Here's how the part is built. I have some questions about the finished solid (model axes, mm). Face numbers are marked on the shaded views. A direction names the side the tool comes from. Give positions to 0.01 mm unless a question says otherwise; leave off trailing zeros. Loops run counter-clockwise (first coordinate to the right, second up) from the corner with the lowest first, then second, coordinate; pieces in that order, holes last. Notation, with made-up numbers: M 78,-20 L 101,-20 A21 ccw 101,-3 Z; hole C 33.5,33.5 d4. An arc over 180 degrees is marked long. Answer as CSV lines item,"result". Start each with the question number.
Item 1: I want a section at B-B on x = -22. List the corners of the cut face in (y, z) for me, plus the area to 3 significant figures.
Item 2: For the marked faces 1 and 2, which set-ups out of +Z, -Z, +X, -X, +Y, -Y let a thin tool reach every point of the face, with its end or its side?
Item 3: I want a section at A-A on z = 20. List the corners of the cut face in (x, y) for me.
Item 4: Will these pins go through, and if not, where does the flat tip stop? P1, Ø19, axis at y = -52, z = 14, coming from the -X side; P2, Ø10, axis at y = 74, z = 34, coming from the -X side; P3, Ø1.5, axis at x = -24, z = 34, coming from the -Y side; P4, Ø1, axis at x = -30, y = 95.5, coming from the -Z side.
Item 5: If I drill on line 1 along Y through (x, z) = (-32.5, 25.5); line 2 along X through (y, z) = (57, 13.5), over which ranges is the centre line in solid material (lowest first)? Write a range as from..to.
Item 6: I want a section at C-C on y = 46.5. List the corners of the cut face in (x, z) for me.
from build123d import *

# Parameters (mm, degrees)
F0_W     = 38.1
F0_H     = 215.9
F0_H_2   = 38.1
F0_W_2   = 63.5
F1_DEPTH = 38.1
F2_SIZE  = 12.7
F3_SIZE  = 31.75
F4_SIZE  = 6.35


with BuildPart() as f1:
    # F0 (on Top) → F1 (new body)
    with BuildSketch(Plane.XY):
        with Locations((0, -19.05)):
            Rectangle(F0_W, F0_H)
        with Locations((0, 107.95)):
            Rectangle(F0_W, F0_H_2)
        with Locations((-50.8, 107.95)):
            Rectangle(F0_W_2, F0_H_2)
    extrude(amount=F1_DEPTH)

    # F2
    f2_edges = [f1.edges().sort_by_distance(p)[0] for p in [
        (-19.05, 88.9, 19.05),
    ]]
    chamfer(f2_edges, length=F2_SIZE)

    # F3
    f3_edges = [f1.edges().sort_by_distance(p)[0] for p in [
        (19.05, 127, 19.05),
    ]]
    chamfer(f3_edges, length=F3_SIZE)

    # F4
    f4_edges = [f1.edges().sort_by_distance(p)[0] for p in [
        (-82.55, 88.9, 19.05),
        (-82.55, 127, 19.05),
    ]]
    chamfer(f4_edges, length=F4_SIZE)


solid = f1.part
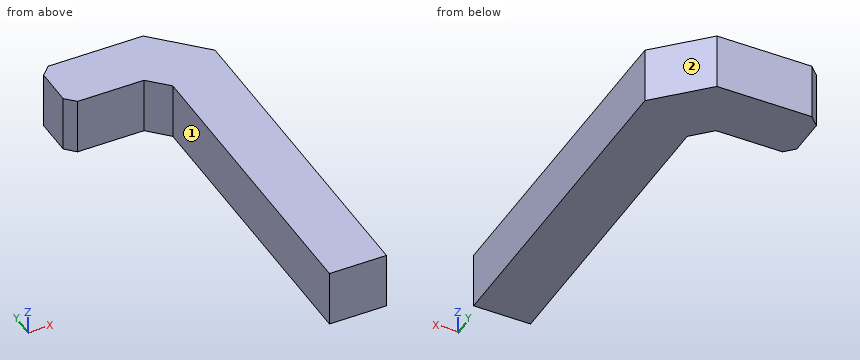
Result:
1,outline,"M 79.15,0 L 127,0 L 127,38.1 L 79.15,38.1 Z"
1,area,"1,820 mm^2"
2,face 1,"+Z, -Z, -X, -Y"
2,face 2,"+Z, -Z, +X, +Y"
3,outline,"M -82.55,95.25 L -76.2,88.9 L -31.75,88.9 L -19.05,76.2 L -19.05,-127 L 19.05,-127 L 19.05,95.25 L -12.7,127 L -76.2,127 L -82.55,120.65 Z"
4,P1,"x = -19.05"
4,P2,"x = -21.85"
4,P3,"y = 80.4"
4,P4,"z = 0"
5,line 1,"88.9..127"
5,line 2,"-19.05..19.05"
6,outline,"M -19.05,0 L 19.05,0 L 19.05,38.1 L -19.05,38.1 Z"
